Source: CAD feature listing. Evaluate the final solid. Frame: model axes, mm. Face numbers are marked on the shaded views. A direction names the side the tool comes from. Round coordinates to 2 decimals unless told otherwise and drop trailing zeros. Order: outer loops, then holes, each group sorted by start corner. A loop starts at its lowest first (then second) coordinate and runs counter-clockwise, first axis right, second up. Notation, with made-up numbers: (-20, -27.75) -> (5, -27.75) arc R26 cw to (5, 10.25) -> close; hole circle Ø5 at (-22.75, 11.25). An arc over 180 degrees is marked (long way). Write item = value, one per line. Start each with the question number.
(1) Cut plane B-B on z = -4.5. Return the cut outline in (x, y) (3 decimals).
(2) Cut plane C-C on x = 22.75. Return the cut outline in (y, z).
(3) Reachability of the marked faces 1 and 2 from +Z, -Z, +X, -X, +Y, -Y: full face, straight path, thin tool, end or side. Return the list, or none.
(4) Cut plane A-A on y = 6.5. Return the cut outline in (x, z), then the cut area to 3 significant figures.
(5) Ray query, line 1 (Y direction, x = 14.5, z = -6.25); line 2 (Y direction, x = 12.5, z = -4.5); line 3 (Z direction, x = 19.75, y = 45.5). Return the intervals inside material, ascending.
(6) Draft query along X for the marked faces 3, 4 and 5. Return one class per face: released by +X, released by -X, zero draft, split by the parting line, or undercut.
(7) Cut plane D-D on y = 44.5. Return the cut outline in (x, z), then the cut area to 3 significant figures.
(8) Contact query for flat-ended pins moving along their axis: pin 1 Ø12 at (x, y) = (15.5, 41) entering from +Z; pin 2 Ø10 at (x, y) = (14.6, 15.54) entering from +Z; pin 3 Ø1.5 at (x, y) = (5.5, 11) entering from -Z; pin 4 Ø1 at (y, z) = (-21, -9) entering from +X. Output: stop coordinate, or through.
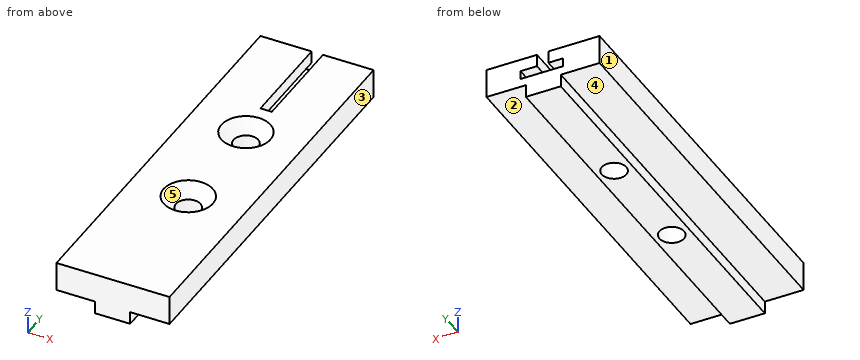
from build123d import *

# Parameters (mm, degrees)
F1_DEPTH       = 25
F2_DEPTH       = 2.1844
F3_DEPTH       = 25.4
F5_D           = 6.35
F5_CSINK_D     = 12.7
F5_CSINK_ANGLE = 90
F6_DEPTH       = 5.08
F7_DEPTH       = 25.4
F8_DEPTH       = 25.4
F9_DEPTH       = 4.064
F11_DEPTH      = 25.4


with BuildPart() as f1:
    # F0 (on Front) → F1 (new body)
    with BuildSketch(Plane.XZ):
        Polygon((29.1909072548, 0), (0, 0), (0, -7.5760227628), (12.1912453324, -7.5760227628), (12.1912453324, -10.8513226733), (18.013689667, -10.8513226733), (18.013689667, -7.5760227628), (29.1909072548, -7.5760227628), align=None)
    extrude(amount=F1_DEPTH)

    # F2 (add): a face of the model
    f2_faces = [f1.faces().sort_by_distance(p)[0] for p in [
        (12.1912453324, -12.5, -9.213672718),
    ]]
    extrude(f2_faces, amount=F2_DEPTH)

    # F3 (add): a face of the model
    f3_faces = [f1.faces().sort_by_distance(p)[0] for p in [
        (14.5334168429, 0, -4.3631968941),
    ]]
    extrude(f3_faces, amount=F3_DEPTH)

    # F5 (through all)
    with Locations(Plane.XY):
        with Locations((14.5954536274, 15.5374109745), (14.5954536274, -13.0615523085)):
            CounterSinkHole(F5_D / 2, F5_CSINK_D / 2, counter_sink_angle=F5_CSINK_ANGLE)

    # F6 (add): a face of the model
    f6_faces = [f1.faces().sort_by_distance(p)[0] for p in [
        (18.013689667, 0.2, -9.213672718),
    ]]
    extrude(f6_faces, amount=F6_DEPTH)

    # F7 (add): a face of the model
    f7_faces = [f1.faces().sort_by_distance(p)[0] for p in [
        (14.9128222173, -25, -4.6688801497),
    ]]
    extrude(f7_faces, amount=F7_DEPTH)

    # F8 (add): a face of the model
    f8_faces = [f1.faces().sort_by_distance(p)[0] for p in [
        (14.9128222173, 25.4, -4.6688801497),
    ]]
    extrude(f8_faces, amount=F8_DEPTH)

    # F9 (cut): a face of the model
    f9_faces = [f1.faces().sort_by_distance(p)[0] for p in [
        (23.093689667, 0.2, -9.213672718),
    ]]
    extrude(f9_faces, amount=-F9_DEPTH, mode=Mode.SUBTRACT)

    # F10 (on face) → F11 (cut)
    with BuildSketch(Plane(origin=(0, 50.8, 0), x_dir=(-1, 0, 0), z_dir=(0, 1, 0))):
        Polygon((-13.2008893415, 0), (-16.1421988159, 0), (-16.1421988159, -3.189817071), (-20.3907564282, -3.189817071), (-20.3907564282, -5.3957989439), (-9.4425510615, -5.3957989439), (-9.4425510615, -3.189817071), (-13.2008893415, -3.189817071), align=None)
    extrude(amount=-F11_DEPTH, mode=Mode.SUBTRACT)


solid = f1.part
Evaluation:
q1.outline = (0, -50.4) -> (29.191, -50.4) -> (29.191, 50.8) -> (20.391, 50.8) -> (20.391, 25.4) -> (9.443, 25.4) -> (9.443, 50.8) -> (0, 50.8) -> close; hole circle Ø6.35 at (14.595, -13.062); hole circle Ø6.35 at (14.595, 15.537)
q2.outline = (-50.4, -7.58) -> (50.8, -7.58) -> (50.8, 0) -> (-50.4, 0) -> close
q3.face_1 = +Z, -Z, -X, +Y, -Y
q3.face_2 = -Z, +X, +Y, -Y
q4.outline = (0, -7.58) -> (10.01, -7.58) -> (10.01, -10.85) -> (19.03, -10.85) -> (19.03, -7.58) -> (29.19, -7.58) -> (29.19, 0) -> (0, 0) -> close
q4.area = 251 mm^2
q5.line_1 = -50.4 to -16.24, -9.89 to 12.36, 18.71 to 50.8
q5.line_2 = -50.4 to -15.45, -10.68 to 13.15, 17.92 to 25.4
q5.line_3 = -7.58 to -5.4, -3.19 to 0
q6.face_3 = released by +X
q6.face_4 = zero draft
q6.face_5 = undercut
q7.outline = (0, -7.58) -> (10.01, -7.58) -> (10.01, -10.85) -> (19.03, -10.85) -> (19.03, -7.58) -> (29.19, -7.58) -> (29.19, 0) -> (16.14, 0) -> (16.14, -3.19) -> (20.39, -3.19) -> (20.39, -5.4) -> (9.44, -5.4) -> (9.44, -3.19) -> (13.2, -3.19) -> (13.2, 0) -> (0, 0) -> close
q7.area = 217 mm^2
q8.pin_1 = 0
q8.pin_2 = -1.34
q8.pin_3 = -7.58
q8.pin_4 = 19.03
